Build history of the part. All positions in model axes, mm. Face numbers are marked on the shaded views. A direction names the side the tool comes from. Coordinates: 2 decimals unless noted, no trailing zeros. Write each loop counter-clockwise with the first axis right and the second up, starting at its lowest first coordinate (ties: lowest second). Pieces come first, ordered by that corner, then holes.
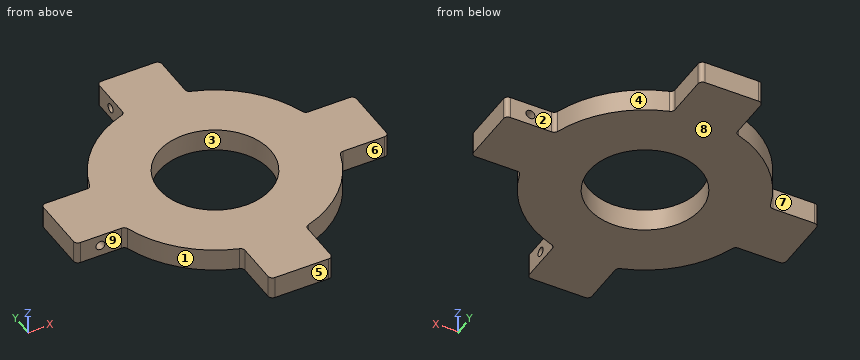
from build123d import *

# Parameters (mm, degrees)
SKETCH1_R           = 12.5
BOSS_EXTRUDE1_DEPTH = 5
SKETCH2_R           = 1
CUT_EXTRUDE1_DEPTH  = 3
CIRPATTERN1_COUNT   = 4
FILLET1_R           = 1
FILLET2_R           = 1


with BuildPart() as part:
    # Sketch1 → Boss-Extrude1 (new body)
    with BuildSketch(Plane.XY):
        with BuildLine():
            Line((35, 7), (24, 7))
            ThreePointArc((24, 7), (17.67766953, 17.67766953), (7, 24))
            Line((7, 24), (7, 35))
            Line((7, 35), (-7, 35))
            Line((-7, 35), (-7, 24))
            ThreePointArc((-7, 24), (-17.67766953, 17.67766953), (-24, 7))
            Line((-24, 7), (-35, 7))
            Line((-35, 7), (-35, -7))
            Line((-35, -7), (-24, -7))
            ThreePointArc((-24, -7), (-17.67766953, -17.67766953), (-7, -24))
            Line((-7, -24), (-7, -35))
            Line((-7, -35), (7, -35))
            Line((7, -35), (7, -24))
            ThreePointArc((7, -24), (17.67766953, -17.67766953), (24, -7))
            Line((24, -7), (35, -7))
            Line((35, -7), (35, 7))
        make_face()
        Circle(SKETCH1_R, mode=Mode.SUBTRACT)
    extrude(amount=BOSS_EXTRUDE1_DEPTH)

    # Sketch2 → Cut-Extrude1 (cut)
    with BuildSketch(Plane(origin=(0, 7, 0), x_dir=(1, 0, 0), z_dir=(0, 1, 0))):
        with Locations((29.5, -2.5)):
            Circle(SKETCH2_R)
    cut_extrude1 = extrude(amount=-CUT_EXTRUDE1_DEPTH, mode=Mode.SUBTRACT)

    # CirPattern1: Cut-Extrude1 ×4 about axis
    cirpattern1_axis = Axis((0, 0, 0), (0, 0, 1))
    for i in range(1, CIRPATTERN1_COUNT):
        add(cut_extrude1.rotate(cirpattern1_axis, i * 360 / CIRPATTERN1_COUNT), mode=Mode.SUBTRACT)

    # Fillet1
    fillet1_edges = [part.edges().sort_by_distance(p)[0] for p in [
        (35, 7, 2.5),
        (35, -7, 2.5),
        (7, -35, 2.5),
        (-7, -35, 2.5),
        (-35, -7, 2.5),
        (-35, 7, 2.5),
        (-7, 35, 2.5),
        (7, 35, 2.5),
    ]]
    fillet(fillet1_edges, radius=FILLET1_R)

    # Fillet2
    fillet2_edges = [part.edges().sort_by_distance(p)[0] for p in [
        (24, 7, 2.5),
        (24, -7, 2.5),
        (7, -24, 2.5),
        (-7, -24, 2.5),
        (-24, -7, 2.5),
        (-24, 7, 2.5),
        (-7, 24, 2.5),
        (7, 24, 2.5),
    ]]
    fillet(fillet2_edges, radius=FILLET2_R)


solid = part.part
(1) 3-axis set-ups, long thin cutter, end or side, ignore diameter. For the marked faces 5, 6, 7, 8 and 9: which of +Z, -Z, +X, -X, +Y, -Y reach the whole face in a straight line?
(2) Two-plate mould, pull along X, no slides. Class the marked faces 1, 2, 3 and 4: pulls with the +X half, pulls with the -X half, needs draft (parallel to the pull), parting line crosses it, or undercut.
(3) Probe L1, parallel to Y at x = 0, z = 3.6; L2, parallel to Z at x = -29.5, y = -6; L3, parallel to X at y = 5.2, z = 2.5. List the from-to ranges inside material, lowest first.
(4) Slice it at A-A, the plane y = 0. List the corners of the cut face in (x, z), and give its area (3 significant figures).
(5) Flat gauge pins, fed straight in: P1, Ø2.5, axis at x = -29, z = 2, coming from the -Y side; P2, Ø1.5, axis at x = -31.5, z = 3.5, coming from the +Y side; P3, Ø1.2, axis at y = 29.5, z = 2.5, coming from the -X side; P4, Ø22.5, axis at x = 0, y = 0, coming from the -Z side. Where does each tip first touch, or does it go through?
(6) Slice it at C-C, the plane y = 29.5. List the corners of the cut face in (x, z).
Results:
1. face 5: +Z, -Z, +X, -X, -Y
1. face 6: +Z, -Z, +X, -Y
1. face 7: +Z, -Z, -X, +Y
1. face 8: -Z, +X, -X, +Y, -Y
1. face 9: +Z, -Z, -X, -Y
2. face 1: pulls with the -X half
2. face 2: needs draft
2. face 3: undercut
2. face 4: pulls with the +X half
3. L1: y = -35 to -12.5, 12.5 to 35
3. L2: z = 0 to 1.5, 3.5 to 5
3. L3: x = -35 to -11.37, 11.37 to 28.5, 30.5 to 35
4. outline: (-35, 0) - (-12.5, 0) - (-12.5, 5) - (-35, 5) - close; (12.5, 0) - (35, 0) - (35, 5) - (12.5, 5) - close
4. area: 225 mm2
5. P1: stops at y = -7
5. P2: stops at y = 7
5. P3: stops at x = -4
5. P4: passes through
6. outline: (-7, 0) - (7, 0) - (7, 5) - (-7, 5) - (-7, 3.5) - (-4, 3.5) - (-4, 1.5) - (-7, 1.5) - close
